Design review of the part shown in the three views and the two pictorial views. Dimensions are in mm from the part's minimum x, y and z. A direction names the side the tool comes from. Round coordinates to 2 decimals unless told otherwise and drop trailing zeros. Write each loop counter-clockwise with the first axis right and the second up, starting at its lowest first coordinate (ties: lowest second). Pieces come first, ordered by that corner, then holes. Notation, with made-up numbers: (-10, -27.5) - (7, -27.5) arc R19 cw to (7, -10.5) - close; hole circle Ø2 at (3, 38). An arc over 180 degrees is marked (long way). Use one line per item in the form item = value.
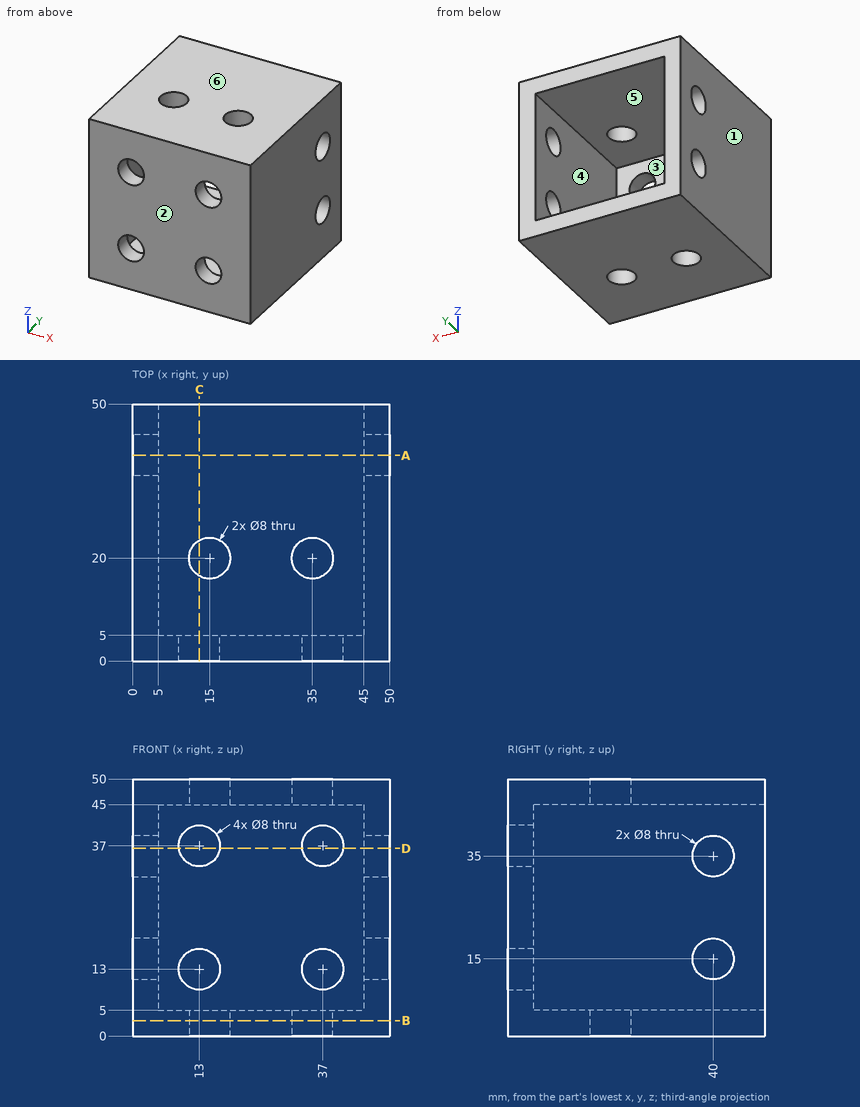
(1) Add section D-D on z = 36.5. Write out the cut boundary in (x, y).
Geometry results:
outline = (0, 0) - (9.03, 0) - (9.03, 5) - (5, 5) - (5, 36.29) - (0, 36.29) - close; (0, 43.71) - (5, 43.71) - (5, 50) - (0, 50) - close; (16.97, 0) - (33.03, 0) - (33.03, 5) - (16.97, 5) - close; (40.97, 0) - (50, 0) - (50, 36.29) - (45, 36.29) - (45, 5) - (40.97, 5) - close; (45, 43.71) - (50, 43.71) - (50, 50) - (45, 50) - close
(2) Add section C-C on x = 13. Write out the cut boundary in (y, z).
Geometry results:
outline = (0, 0) - (16.54, 0) - (16.54, 5) - (5, 5) - (5, 9) - (0, 9) - close; (0, 17) - (5, 17) - (5, 33) - (0, 33) - close; (0, 41) - (5, 41) - (5, 45) - (16.54, 45) - (16.54, 50) - (0, 50) - close; (23.46, 0) - (50, 0) - (50, 5) - (23.46, 5) - close; (23.46, 45) - (50, 45) - (50, 50) - (23.46, 50) - close
(3) Insertion check: P1, Ø4, axis at x = 24.5, z = 40, coming from the +Y side. The pin has a flat end and moves straight along its axis. Give the tip position at first contact, or say it passes through.
Geometry results:
P1 = 5
(4) Add section B-B on z = 3. Write out the cut boundary in (x, y), then the cut area to 3 significant figures.
Geometry results:
outline = (0, 0) - (50, 0) - (50, 50) - (0, 50) - close; hole circle Ø8 at (15, 20); hole circle Ø8 at (35, 20)
area = 2,400 mm2
(5) To check wall thickness, follow L1, parallel to Z at x = 1.2, y = 40; L2, parallel to Y at x = 35, z = 46; L3, parallel to Z at x = 17, y = 16.5. State the ranges of each line that lie inside material, in increasing order.
Geometry results:
L1 = 0 to 11, 19 to 31, 39 to 50
L2 = 0 to 16, 24 to 50
L3 = 0 to 5, 45 to 50
(6) Add section A-A on y = 40. Write out the cut boundary in (x, z), then the cut area to 3 significant figures.
Geometry results:
outline = (0, 0) - (50, 0) - (50, 11) - (45, 11) - (45, 5) - (5, 5) - (5, 11) - (0, 11) - close; (0, 19) - (5, 19) - (5, 31) - (0, 31) - close; (0, 39) - (5, 39) - (5, 45) - (45, 45) - (45, 39) - (50, 39) - (50, 50) - (0, 50) - close; (45, 19) - (50, 19) - (50, 31) - (45, 31) - close
area = 740 mm2
(7) Machinability: for the marked faces 5 and 6, which of the approach directions +Z, -Z, +X, -X, +Y, -Y give a long, thin tool a straight path to every point of the face, cutting with its end or side? Answer none if there is none.
Geometry results:
face_5 = +Y
face_6 = +Z, +X, -X, +Y, -Y
(8) The part is to be moulded in two halves that separate along X. For the marked faces 1, 2, 3 and 4, say which applies: +X half, -X half, draft (parallel to the pull), parting line (faces both ways), or undercut.
Geometry results:
face_1 = -X half
face_2 = draft
face_3 = undercut
face_4 = undercut
